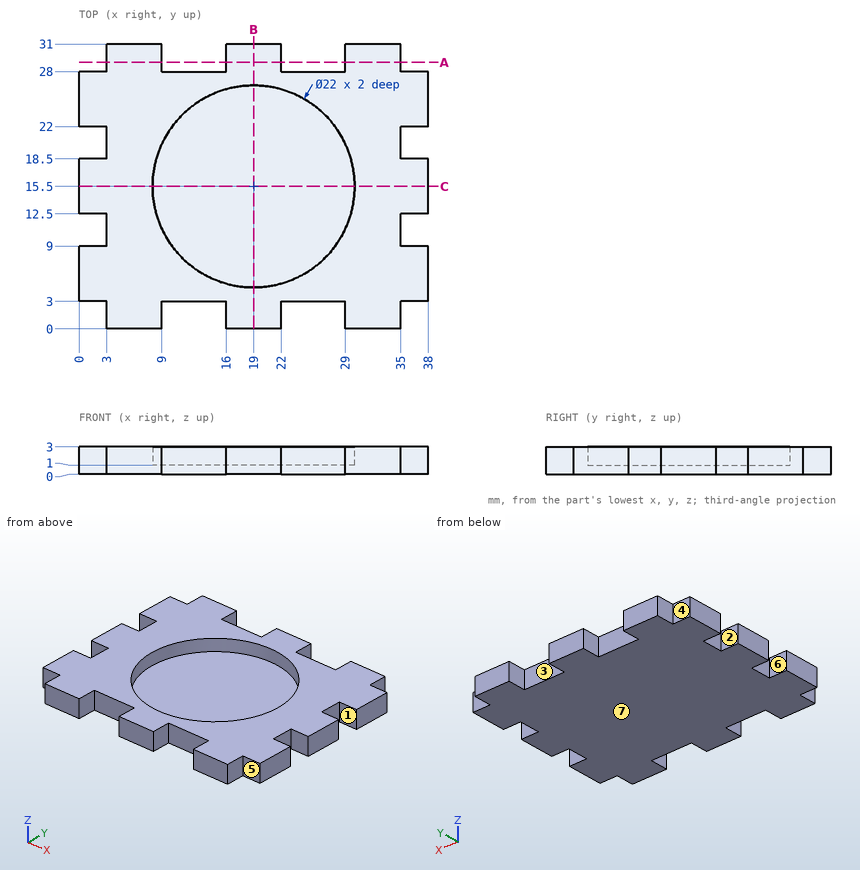
Could you check a few things on this drawing? It's one solid part, dimensions in mm from its lowest x, y, z. A direction names the side the tool comes from. Coordinates: 2 decimals unless noted, no trailing zeros. Order: outer loops, then holes, each group sorted by start corner. A loop starts at its lowest first (then second) coordinate and runs counter-clockwise, first axis right, second up.
1) Imagine slicing it at C-C on y = 15.5. List the corners of the cut face in (x, z) for me, and give its area (3 significant figures).
2) Imagine slicing it at B-B on x = 19. List the corners of the cut face in (y, z) for me.
3) Will these pins go through, and if not, where does the flat tip stop? pin 1 (0.9 mm diameter, centred on x = 24.5, z = 1, fed in from +Y); pin 2 (0.9 mm diameter, centred on x = 2, z = 1, fed in from -Y); pin 3 (1.5 mm diameter, centred on y = 29.5, z = 1.5, fed in from -X).
4) We'd pull the mould along Y, two halves only. Please class the marked faces 5, 6 and 7: +Y half, -Y half, draft (parallel to the pull), parting line (faces both ways), or undercut.
5) Which directions (+Z, -Z, +X, -X, +Y, -Y) give clear straight access to the entire face, cutting with the end or side of a thin tool? Please do the marked faces 1, 2, 3 and 4.
6) I need wall thicknesses on line 1 (X direction, y = 2.5, z = 2.85); line 2 (X direction, y = 15.5, z = 1.9); line 3 (Y direction, x = 19, z = 1.8). Which ranges of each line are inside material? Lowest first, please.
7) Imagine slicing it at A-A on y = 29. List the corners of the cut face in (x, z) for me, and give its area (3 significant figures).
Response values:
1. outline: (0, 0) - (38, 0) - (38, 3) - (30, 3) - (30, 1) - (8, 1) - (8, 3) - (0, 3) - close
1. area: 70.0 mm2
2. outline: (0, 0) - (31, 0) - (31, 3) - (26.5, 3) - (26.5, 1) - (4.5, 1) - (4.5, 3) - (0, 3) - close
3. pin 1: stops at y = 28
3. pin 2: stops at y = 3
3. pin 3: stops at x = 3
4. face 5: -Y half
4. face 6: undercut
4. face 7: draft
5. face 1: +Z, -Z, +X
5. face 2: +Z, -Z, -X
5. face 3: +Z, -Z, +Y
5. face 4: +Z, -Z, -X, +Y
6. line 1: x = 3 to 9, 16 to 22, 29 to 35
6. line 2: x = 0 to 8, 30 to 38
6. line 3: y = 0 to 4.5, 26.5 to 31
7. outline: (3, 0) - (9, 0) - (9, 3) - (3, 3) - close; (16, 0) - (22, 0) - (22, 3) - (16, 3) - close; (29, 0) - (35, 0) - (35, 3) - (29, 3) - close
7. area: 54.0 mm2
